Can you work these out from the model? Positions are in its coordinate system, mm. A direction names the side the tool comes from. Give positions to 0.01 mm unless a question says otherwise; leave off trailing zeros. Write each loop counter-clockwise with the first axis right and the second up, starting at its lowest first coordinate (ties: lowest second). Pieces come first, ordered by that corner, then holes.
from build123d import *

# Parameters (mm, degrees)
SKETCH1_W           = 47.6758
SKETCH1_H           = 68.834
BOSS_EXTRUDE1_DEPTH = 7.112
SKETCH11_W          = 47.6758
SKETCH11_H          = 7.112
BOSS_EXTRUDE2_DEPTH = 30.2768
FILLET3_R           = 9.9314
FILLET6_R           = 4.3688
SHELL1_T            = -0.4064


with BuildPart() as part:
    # Sketch1 → Boss-Extrude1 (new body)
    with BuildSketch(Plane.XY):
        with Locations((0, -34.417)):
            Rectangle(SKETCH1_W, SKETCH1_H)
    extrude(amount=-BOSS_EXTRUDE1_DEPTH)

    # Sketch11 → Boss-Extrude2 (add)
    with BuildSketch(Plane(origin=(0, 0, 0), x_dir=(1, 0, 0), z_dir=(0, 1, 0))):
        with Locations((0, 3.556)):
            Rectangle(SKETCH11_W, SKETCH11_H)
    extrude(amount=BOSS_EXTRUDE2_DEPTH)

    # Fillet3
    fillet3_edges = [part.edges().sort_by_distance(p)[0] for p in [
        (-23.8379, 30.2768, -3.556),
        (23.8379, 30.2768, -3.556),
        (23.8379, -68.834, -3.556),
        (-23.8379, -68.834, -3.556),
    ]]
    fillet(fillet3_edges, radius=FILLET3_R)

    # Fillet6
    fillet6_edges = [part.edges().sort_by_distance(p)[0] for p in [
        (-23.8379, -19.2786, -7.112),
        (-20.929060287, -65.925160287, -7.112),
        (0, -68.834, -7.112),
        (23.8379, -19.2786, -7.112),
        (-20.929060287, 27.367960287, -7.112),
        (0, 30.2768, -7.112),
        (20.929060287, 27.367960287, -7.112),
    ]]
    fillet(fillet6_edges, radius=FILLET6_R)

    # Shell1
    shell1_openings = [part.faces().sort_by_distance(p)[0] for p in [
        (0, -19.2786, 0),
    ]]
    offset(amount=SHELL1_T, openings=shell1_openings, kind=Kind.INTERSECTION)


solid = part.part
(1) Imagine slicing it at A-A, the plane x = 11. Write out the boundary of the cut face in (y, z).
Returned:
outline: (-68.83, -2.74) arc R4.37 ccw to (-64.47, -7.11) - (25.91, -7.11) arc R4.37 ccw to (30.28, -2.74) - (30.28, 0) - (29.87, 0) - (29.87, -2.74) arc R3.96 cw to (25.91, -6.71) - (-64.47, -6.71) arc R3.96 cw to (-68.43, -2.74) - (-68.43, 0) - (-68.83, 0) - close
(2) Imagine slicing it at B-B, the plane y = 1. Write out the boundary of the cut face in (x, z).
Returned:
outline: (-23.84, -2.74) arc R4.37 ccw to (-19.47, -7.11) - (19.47, -7.11) arc R4.37 ccw to (23.84, -2.74) - (23.84, 0) - (23.43, 0) - (23.43, -2.74) arc R3.96 cw to (19.47, -6.71) - (-19.47, -6.71) arc R3.96 cw to (-23.43, -2.74) - (-23.43, 0) - (-23.84, 0) - close
(3) For faces 1 (the face through (-0.195, 28.74, -5.514)), 2 (the face through (-21.006, 27.29, -1.391)), which set-ups out of +Z, -Z, +X, -X, +Y, -Y let a thin tool reach every point of the face, with its end or its side?
Returned:
face 1: +Z
face 2: +Z, -Z, -X, +Y
(4) Imagine slicing it at C-C, the plane z = -4.75. Write out the boundary of the cut face in (x, y).
Returned:
outline: (-23.35, -58.9) arc R9.44 ccw to (-13.91, -68.35) - (13.91, -68.35) arc R9.44 ccw to (23.35, -58.9) - (23.35, 20.35) arc R9.44 ccw to (13.91, 29.79) - (-13.91, 29.79) arc R9.44 ccw to (-23.35, 20.35) - close; hole (-22.89, -58.9) arc R8.98 ccw to (-13.91, -67.88) - (13.91, -67.88) arc R8.98 ccw to (22.89, -58.9) - (22.89, 20.35) arc R8.98 ccw to (13.91, 29.32) - (-13.91, 29.32) arc R8.98 ccw to (-22.89, 20.35) - close
(5) If we mould it in two halves opening along Y, with no side actions, what happens to faces 3 (the face through (0.195, -67.588, -5.798)), 4 (the face through (-0.19, 29.03, -5.8)), 5 (the face through (22.302, -18.724, -5.514))? For each: +Y half, -Y half, draft (parallel to the pull), parting line (faces both ways), or undercut.
Returned:
face 3: -Y half
face 4: +Y half
face 5: undercut
(6) If I drill on L1, parallel to Y at x = -7, z = -1.75; L2, parallel to X at y = -20.5, z = -2.75; L3, parallel to Z at x = 14, y = -8, over which ranges is the centre line in solid material (lowest first)?
Returned:
L1: y = -68.83 to -68.43, 29.87 to 30.28
L2: x = -23.84 to -23.43, 23.43 to 23.84
L3: z = -7.11 to -6.71
(7) Will these pins go through, and if not, where does the flat tip stop? P1, Ø4, axis at x = 4, y = -42.5, coming from the +Z side; P2, Ø1, axis at x = 4.5, z = -4.5, coming from the +Y side; P3, Ø2, axis at x = -5, z = -5.5, coming from the -Y side.
Returned:
P1: stops at z = -6.71
P2: stops at y = 30.09
P3: stops at y = -68.47
